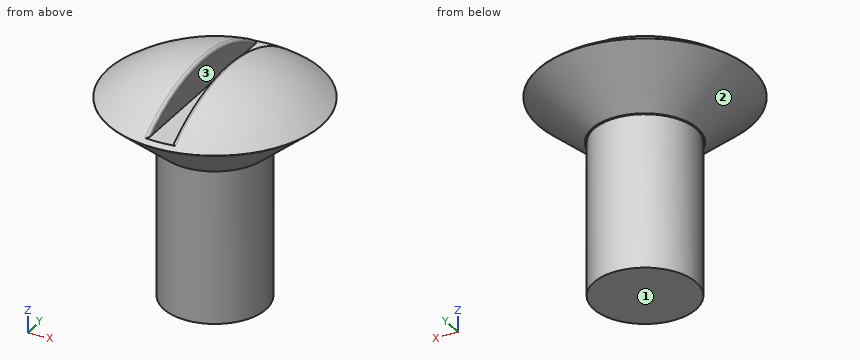
```python
from build123d import *

# Parameters (mm, degrees)
SKETCH1_R           = 3.5433
BOSS_EXTRUDE1_DEPTH = 0.01
DOME1_FACE_RADIUS   = 3.5433
DOME1_HEIGHT        = 1.2
SKETCH2_R           = 3.5433
BOSS_EXTRUDE2_DEPTH = 1.5
BOSS_EXTRUDE2_TAPER = 50
SKETCH3_R           = 1.7
BOSS_EXTRUDE3_DEPTH = 5.1
SKETCH4_W           = 0.8
SKETCH4_H           = 7.6
CUT_EXTRUDE1_DEPTH  = 3
FILLET3_R           = 0.1


with BuildPart() as part:
    # Sketch1 → Boss-Extrude1 (new body)
    with BuildSketch(Plane.XY):
        with Locations(Location((0, 0, 0), (0, 0, 180))):
            Circle(SKETCH1_R)
    extrude(amount=BOSS_EXTRUDE1_DEPTH)

    # Dome1: a dome of height H over a round flat face of radius A is a cap of a sphere of radius (A * A + H * H) / (2 * H)
    dome1_r = (DOME1_FACE_RADIUS * DOME1_FACE_RADIUS + DOME1_HEIGHT * DOME1_HEIGHT) / (2 * DOME1_HEIGHT)
    dome1_base = Plane((0, 0, 0.01), z_dir=(0, 0, 1))
    with Locations(dome1_base.offset(DOME1_HEIGHT - dome1_r)):
        dome1_ball = Sphere(dome1_r, mode=Mode.PRIVATE)
    add(split(dome1_ball, bisect_by=dome1_base, keep=Keep.TOP, mode=Mode.PRIVATE))

    # Sketch2 → Boss-Extrude2 (add)
    with BuildSketch(Plane(origin=(0, 0, 0), x_dir=(-1, 0, 0), z_dir=(0, 0, -1))):
        Circle(SKETCH2_R)
    extrude(amount=BOSS_EXTRUDE2_DEPTH, taper=BOSS_EXTRUDE2_TAPER)

    # Sketch3 → Boss-Extrude3 (add)
    with BuildSketch(Plane(origin=(0, 0, -1.5), x_dir=(-1, 0, 0), z_dir=(0, 0, -1))):
        Circle(SKETCH3_R)
    extrude(amount=BOSS_EXTRUDE3_DEPTH)

    # Sketch4 → Cut-Extrude1 (cut)
    with BuildSketch(Plane.XY.offset(0.133904)):
        Rectangle(SKETCH4_W, SKETCH4_H)
    extrude(amount=CUT_EXTRUDE1_DEPTH, mode=Mode.SUBTRACT)

    # Fillet3
    fillet3_edges = [part.edges().sort_by_distance(p)[0] for p in [
        (0.4, -1.757880439, 0.924318226),
        (-0.4, 0, 1.196264613),
    ]]
    fillet(fillet3_edges, radius=FILLET3_R)


solid = part.part
```
CAD build for the part. Positions are in the model's coordinates, mm. Face numbers are marked on the shaded views. Coordinates: 2 decimals unless noted, no trailing zeros. Order: outer loops, then holes, each group sorted by start corner. A loop starts at its lowest first (then second) coordinate and runs counter-clockwise, first axis right, second up. Notation, with made-up numbers: (7, 55.25) - (26, 55.25) arc R31 ccw to (26, 91.25) - close; hole circle Ø8 at (54, 26.25). An arc over 180 degrees is marked (long way). Use a Markdown table: item, result. Add a question column.
(1) Flat gauge pins, fed straight in: pin 1 (0.5 mm diameter, centred on x = 0, y = -1.5, fed in from +Z); pin 2 (4 mm diameter, centred on x = 2, y = 1.5, fed in from +Z); pin 3 (0.5 mm diameter, centred on y = -1, z = 0.5, fed in from -X). Where does each tip first touch, or does it go through?
(2) Saw through at B-B (z = -2.75). Give the cut face in (x, y).
(3) Pull direction X, two halves, no side cores. Call the marked faces 1, 2 and 3: +X half, -X half, draft (parallel to the pull), parting line (faces both ways), or undercut.
(4) Drill centre lines: line 1 along Z through (x, y) = (0.25, 1); line 2 along X through (y, z) = (1.25, -0.5); line 3 along Z through (x, y) = (1.5, 1). Where is each one in solid material? Low to high. Write a range as [from, to].
Solved:
| question | item | result |
|---|---|---|
| 1 | pin 1 | stops at z = 0.13 |
| 1 | pin 2 | stops at z = 1.19 |
| 1 | pin 3 | stops at x = -3.05 |
| 2 | outline | circle Ø3.4 at (0, 0) |
| 3 | face 1 | draft |
| 3 | face 2 | parting line |
| 3 | face 3 | undercut |
| 4 | line 1 | z = [-6.6, 0.13] |
| 4 | line 2 | x = [-2.67, 2.67] |
| 4 | line 3 | z = [-1.46, 0.92] |
